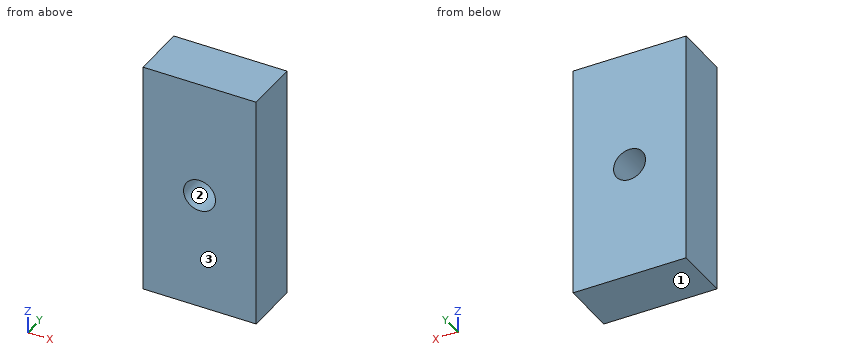
from build123d import *

# Parameters (mm, degrees)
SKETCH1_W             = 8.001
SKETCH1_H             = 16.5354
BOSS_EXTRUDE1_DEPTH   = 3.937
F_4_40_TAPPED_HOLE1_D = 2.2606


with BuildPart() as part:
    # Sketch1 → Boss-Extrude1 (new body)
    with BuildSketch(Plane(origin=(0, 0, 0), x_dir=(1, 0, 0), z_dir=(0, 1, 0))):
        Rectangle(SKETCH1_W, SKETCH1_H)
    extrude(amount=BOSS_EXTRUDE1_DEPTH)

    # #4-40 Tapped Hole1 (through all)
    with Locations(Plane(origin=(0, 3.937, 0), x_dir=(1, 0, 0), z_dir=(0, 1, 0))):
        with Locations((0, 0)):
            Hole(F_4_40_TAPPED_HOLE1_D / 2)


solid = part.part
The listing builds one solid part. Answer for the finished solid, in the listing's coordinates (mm). Face numbers are marked on the shaded views. Coordinates: 2 decimals unless noted, no trailing zeros. Order: outer loops, then holes, each group sorted by start corner. A loop starts at its lowest first (then second) coordinate and runs counter-clockwise, first axis right, second up. Notation, with made-up numbers: (-38.5, 66.5) -> (8.5, 66.5) arc R12 ccw to (8.5, 84.5) -> close; hole circle Ø5 at (49.25, 54.5). An arc over 180 degrees is marked (long way). Answer in a Markdown table with one row per item. Add a question column.
Item 1: Find section A-A (x = 0). Write down the section's boundary in (y, z).
Item 2: Find section B-B (z = 0). Write down the section's boundary in (x, y), then the cut area to 3 significant figures.
Item 3: Find the intervals of material crossed by L1, parallel to Z at x = 0, y = 1.3; L2, parallel to Z at x = -0.75, y = 2.65; L3, parallel to X at y = 1.55, z = -0.25, in increasing order. Write a range as from..to.
Item 4: Determine the mould class of the marked faces 1, 2 and 3 for opening direction Z: +Z half, -Z half, draft (parallel to the pull), parting line (faces both ways), or undercut.
Item 5: Find section C-C (y = 3.5). Write down the section's boundary in (x, z), then the cut area to 3 significant figures.
Result set:
| question | item | result |
|---|---|---|
| 1 | outline | (0, -8.27) -> (3.94, -8.27) -> (3.94, -1.13) -> (0, -1.13) -> close; (0, 1.13) -> (3.94, 1.13) -> (3.94, 8.27) -> (0, 8.27) -> close |
| 2 | outline | (-4, 0) -> (-1.13, 0) -> (-1.13, 3.94) -> (-4, 3.94) -> close; (1.13, 0) -> (4, 0) -> (4, 3.94) -> (1.13, 3.94) -> close |
| 2 | area | 22.6 mm² |
| 3 | L1 | z = -8.27..-1.13, 1.13..8.27 |
| 3 | L2 | z = -8.27..-0.85, 0.85..8.27 |
| 3 | L3 | x = -4..-1.1, 1.1..4 |
| 4 | face 1 | -Z half |
| 4 | face 2 | undercut |
| 4 | face 3 | draft |
| 5 | outline | (-4, -8.27) -> (4, -8.27) -> (4, 8.27) -> (-4, 8.27) -> close; hole circle Ø2.26 at (0, 0) |
| 5 | area | 128 mm² |
